```python
from build123d import *

# Parameters (mm, degrees)
SKETCH1_R             = 100
BOSS_EXTRUDE1_DEPTH   = 8
SKETCH2_R             = 17.5
CUT_EXTRUDE1_DEPTH    = 142.647449677
SKETCH3_R             = 9.009876889
CUT_EXTRUDE2_DEPTH    = 7.269341
CIRPATTERN1_START     = 0.730659227
CIRPATTERN1_OUTLINE_R = 9.009876889
CIRPATTERN1_DEPTH     = 7.269340773


# Read off the part's stored shape, not the designer's step: CirPattern1
with BuildPart() as part:
    # Sketch1 → Boss-Extrude1 (new body)
    with BuildSketch(Plane(origin=(0, 0, 0), x_dir=(1, 0, 0), z_dir=(0, 1, 0))):
        with Locations(Location((0, 0, 0), (0, 0, 270))):
            Circle(SKETCH1_R)
    extrude(amount=BOSS_EXTRUDE1_DEPTH)

    # Sketch2 → Cut-Extrude1 (cut, through all)
    with BuildSketch(Plane(origin=(0, 0, 0), x_dir=(1, 0, 0), z_dir=(0, 1, 0))):
        with Locations(Location((0, 0, 0), (0, 0, 270))):
            Circle(SKETCH2_R)
    extrude(amount=CUT_EXTRUDE1_DEPTH, mode=Mode.SUBTRACT)

    # Sketch3 → Cut-Extrude2 (cut)
    with BuildSketch(Plane(origin=(0, 8, 0), x_dir=(1, 0, 0), z_dir=(0, 1, 0))):
        with Locations(Location((-42.948020952, 0, 0), (0, 0, 270))):
            Circle(SKETCH3_R)
    extrude(amount=-CUT_EXTRUDE2_DEPTH, mode=Mode.SUBTRACT)

    # CirPattern1 outline → CirPattern1 (cut)
    with BuildSketch(Plane(origin=(0, 0, 0), x_dir=(1, 0, 0), z_dir=(0, 1, 0)).offset(CIRPATTERN1_START)):
        with Locations((21.474010476, 37.194077186)):
            Circle(CIRPATTERN1_OUTLINE_R)
        with Locations((21.474010476, -37.194077186)):
            Circle(CIRPATTERN1_OUTLINE_R)
    extrude(amount=CIRPATTERN1_DEPTH, mode=Mode.SUBTRACT)


solid = part.part
```
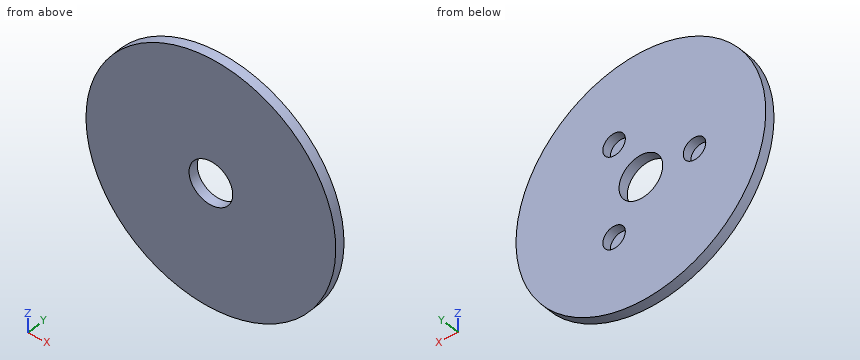
Geometry check sheet. Reference: the model listing, model coordinates, mm. Give positions to 0.01 mm unless a question says otherwise; leave off trailing zeros. Order: outer loops, then holes, each group sorted by start corner. A loop starts at its lowest first (then second) coordinate and runs counter-clockwise, first axis right, second up. Notation, with made-up numbers: (-38, 10.25) -> (-7, 10.25) arc R25 ccw to (-7, 34.25) -> close; hole circle Ø10 at (20.5, -10). An arc over 180 degrees is marked (long way). Write each question's results on one line, items separated by ' | '. Start each with the question number.
(1) Gauge pin test, flat ends, axial feed: P1, Ø4, axis at x = 72.5, y = 6, coming from the +Z side; P2, Ø1.5, axis at x = -37, z = 3, coming from the +Y side; P3, Ø1.5, axis at x = -5, y = 2.5, coming from the -Z side. Record the tip position at first contact, or that the pin passes through.
(2) Scan lines: line 1 (X direction, y = 4.75, z = 0); line 2 (X direction, y = 4.5, z = 8); line 3 (Z direction, x = 26.5, y = 4.75). Record each from-to range of solid material in increasing order.
(3) Sectioned sample at C-C (x = -37). Enter the section's corners in (y, z).
(4) Sectioned sample at A-A (z = 0). Enter the section's corners in (x, y), plus the area to 3 significant figures.
(5) Sectioned sample at B-B (x = 0). Enter the section's corners in (y, z).
(6) Sectioned sample at D-D (y = 2.25). Enter the section's corners in (x, z), plus the area to 3 significant figures.
Answer below:
1) P1: z = 70.92 | P2: y = 0.73 | P3: z = -99.91
2) line 1: -100 to -51.96, -33.94 to -17.5, 17.5 to 100 | line 2: -99.68 to -47.09, -38.8 to -15.56, 15.56 to 99.68 | line 3: -96.42 to -44.67, -29.72 to 29.72, 44.67 to 96.42
3) outline: (0, -92.9) -> (8, -92.9) -> (8, -6.77) -> (0.73, -6.77) -> (0.73, 6.77) -> (8, 6.77) -> (8, 92.9) -> (0, 92.9) -> close
4) outline: (-100, 0) -> (-17.5, 0) -> (-17.5, 8) -> (-33.94, 8) -> (-33.94, 0.73) -> (-51.96, 0.73) -> (-51.96, 8) -> (-100, 8) -> close; (17.5, 0) -> (100, 0) -> (100, 8) -> (17.5, 8) -> close | area: 1,190 mm2
5) outline: (0, -100) -> (8, -100) -> (8, -17.5) -> (0, -17.5) -> close; (0, 17.5) -> (8, 17.5) -> (8, 100) -> (0, 100) -> close
6) outline: circle Ø200 at (0, 0); hole circle Ø18.02 at (-42.95, 0); hole circle Ø35 at (0, 0); hole circle Ø18.02 at (21.47, -37.19); hole circle Ø18.02 at (21.47, 37.19) | area: 29,700 mm2
